Check sheet for the modelled part. Datum: model origin and axes. Units: mm. Face numbers are marked on the shaded views. A direction names the side the tool comes from. Give positions to 0.01 mm unless a question says otherwise; leave off trailing zeros. Loops run counter-clockwise (first coordinate to the right, second up) from the corner with the lowest first, then second, coordinate; pieces in that order, holes last. Notation, with made-up numbers: M -22,5.5 L -1,5.5 A5 ccw -1,14.5 Z; hole C 7.25,-1 d5. An arc over 180 degrees is marked long. Use one line per item in the form item = value.
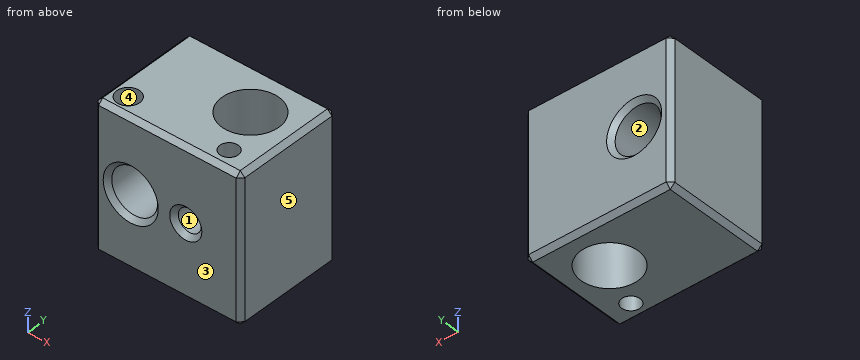
from build123d import *

# Parameters (mm, degrees)
SKETCH1_W                       = 16
SKETCH1_H                       = 16
BOSS_EXTRUDE1_DEPTH             = 12
SKETCH2_R                       = 3.1
SKETCH2_R_2                     = 1
CUT_EXTRUDE1_DEPTH              = 17
F_2_5_2_5_DIAMETER_HOLE1_D      = 2.5
F_2_5_2_5_DIAMETER_HOLE1_DEPTH  = 4.5
TAP_DRILL_FOR_M6X1_0_TAP1_D     = 5
TAP_DRILL_FOR_M3X0_5_TAP1_D     = 2.5
TAP_DRILL_FOR_M3X0_5_TAP1_DEPTH = 6.999
TAP_DRILL_FOR_M3X0_5_TAP1_TIP   = 0.751075774
CHAMFER1_SIZE                   = 0.5


with BuildPart() as part:
    # Sketch1 → Boss-Extrude1 (new body)
    with BuildSketch(Plane(origin=(0, 0, 0), x_dir=(1, 0, 0), z_dir=(0, 1, 0))):
        Rectangle(SKETCH1_W, SKETCH1_H)
    extrude(amount=BOSS_EXTRUDE1_DEPTH)

    # Sketch2 → Cut-Extrude1 (cut, through all)
    with BuildSketch(Plane.XY.offset(8)):
        with Locations((3, 7)):
            Circle(SKETCH2_R)
        with Locations((5, 2)):
            Circle(SKETCH2_R_2)
    extrude(amount=-CUT_EXTRUDE1_DEPTH, mode=Mode.SUBTRACT)

    # Ø2.5 (2.5) Diameter Hole1
    with Locations(Plane.XY.offset(8)):
        with Locations((-6, 2)):
            Hole(F_2_5_2_5_DIAMETER_HOLE1_D / 2, depth=F_2_5_2_5_DIAMETER_HOLE1_DEPTH)

    # Tap Drill for M6x1.0 Tap1 (through all)
    with Locations(Plane(origin=(0, 12, 0), x_dir=(1, 0, 0), z_dir=(0, 1, 0))):
        with Locations((-4, 0)):
            Hole(TAP_DRILL_FOR_M6X1_0_TAP1_D / 2)

    # Tap Drill for M3x0.5 Tap1
    with Locations(Plane(origin=(0, 0, 0), x_dir=(-1, 0, 0), z_dir=(0, -1, 0))):
        with Locations((-2, 0)):
            Hole(TAP_DRILL_FOR_M3X0_5_TAP1_D / 2, depth=TAP_DRILL_FOR_M3X0_5_TAP1_DEPTH)
            with Locations((0, 0, -(TAP_DRILL_FOR_M3X0_5_TAP1_DEPTH + TAP_DRILL_FOR_M3X0_5_TAP1_TIP / 2))):  # 118° drill point
                Cone(0, TAP_DRILL_FOR_M3X0_5_TAP1_D / 2, TAP_DRILL_FOR_M3X0_5_TAP1_TIP, mode=Mode.SUBTRACT)

    # Chamfer1
    chamfer1_edges = [part.edges().sort_by_distance(p)[0] for p in [
        (0, 12, -8),
        (-8, 12, 0),
        (-1.5, 12, 0),
        (-1.5, 0, 0),
        (0.75, 0, 0),
        (0, 12, 8),
        (-8, 0, 0),
        (0, 0, -8),
        (8, 0, 0),
        (0, 0, 8),
        (8, 12, 0),
        (-8, 6, 8),
        (-8, 6, -8),
        (8, 6, -8),
        (8, 6, 8),
    ]]
    chamfer(chamfer1_edges, length=CHAMFER1_SIZE)


solid = part.part
1) Section check B-B (y = 10.5). Record the cut outline in (x, z).
Evaluation:
outline = M -8,-7.5 L -7.5,-8 L 7.5,-8 L 8,-7.5 L 8,7.5 L 7.5,8 L -7.5,8 L -8,7.5 Z; hole C -4,0 d5
2) Section check D-D (x = 4.5). Record the cut outline in (y, z), then the cut area to 3 significant figures.
Evaluation:
outline = M 0,-7.5 L 0.5,-8 L 1.13,-8 L 1.13,8 L 0.5,8 L 0,7.5 Z; M 2.87,-8 L 4.29,-8 L 4.29,8 L 2.87,8 Z; M 9.71,-8 L 11.5,-8 L 12,-7.5 L 12,7.5 L 11.5,8 L 9.71,8 Z
area = 77.0 mm^2
3) Release check for a two-part mould opening along Y. For the marked faces 3, 4 and 5 record: pulls with the +Y half, pulls with the -Y half, needs draft (parallel to the pull), parting line crosses it, or undercut.
Evaluation:
face_3 = pulls with the -Y half
face_4 = undercut
face_5 = needs draft
4) Section check A-A (x = -4). Record the cut outline in (y, z), then the cut area to 3 significant figures.
Evaluation:
outline = M 0,-7.5 L 0.5,-8 L 11.5,-8 L 12,-7.5 L 12,-3 L 11.5,-2.5 L 0.5,-2.5 L 0,-3 Z; M 0,3 L 0.5,2.5 L 11.5,2.5 L 12,3 L 12,7.5 L 11.5,8 L 0.5,8 L 0,7.5 Z
area = 131 mm^2
5) Set-up check for the marked faces 1 and 2: record each of +Z, -Z, +X, -X, +Y, -Y from which the full face is reachable in a straight line by a thin tool's end or side.
Evaluation:
face_1 = -Y
face_2 = +Y, -Y
6) Scan lines: line 1 (Z direction, x = 1.25, y = 1.5); line 2 (X direction, y = 5.25, z = 0.25); line 3 (Z direction, x = 2, y = 1.65). Record each from-to range of solid material in increasing order.
Evaluation:
line_1 = -8 to -1, 1 to 8
line_2 = -8 to -6.49, -1.51 to 0.44, 5.56 to 8
line_3 = -8 to -1.25, 1.25 to 8
7) Section check C-C (z = 0). Record the cut outline in (x, y).
Evaluation:
outline = M -8,0.5 L -7.5,0 L -7,0 L -6.5,0.5 L -6.5,11.5 L -7,12 L -7.5,12 L -8,11.5 Z; M -1.5,0.5 L -1,0 L 0.25,0 L 0.75,0.5 L 0.75,4.87 A3.1 cw long 3.25,3.91 L 3.25,0.5 L 3.75,0 L 7.5,0 L 8,0.5 L 8,11.5 L 7.5,12 L -1,12 L -1.5,11.5 Z; hole C 5,2 d2
